Print and shaded views of the part. All mm, measured from the part's lowest x, y and z. A direction names the side the tool comes from. Give positions to 0.01 mm unless a question says otherwise; leave off trailing zeros. Loops run counter-clockwise (first coordinate to the right, second up) from the corner with the lowest first, then second, coordinate; pieces in that order, holes last. Notation, with made-up numbers: (66.25, 63) -> (78.25, 63) arc R25 cw to (78.25, 92) -> close; hole circle Ø6 at (32, 64). An arc over 180 degrees is marked (long way). Answer as a JSON object with one key per item and string values. Group by question number.
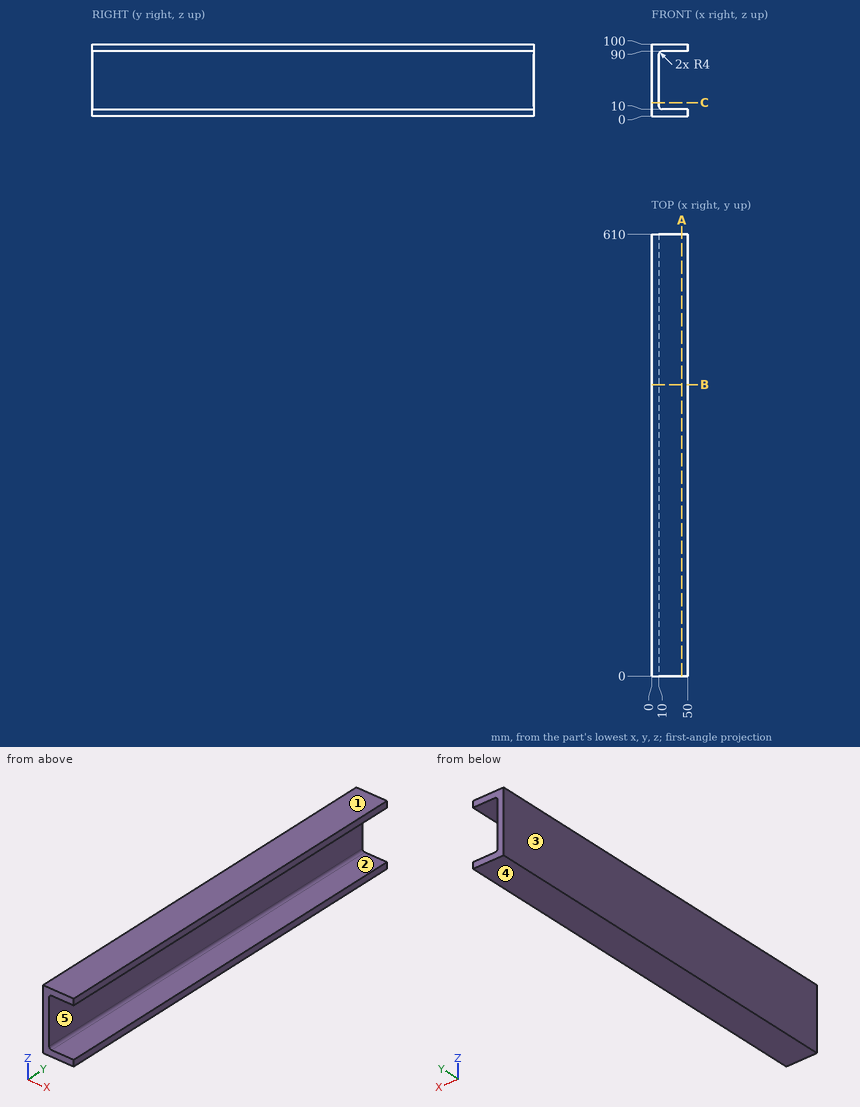
(1) Saw through at C-C on z = 19. List the corners of the cut face in (x, y).
(2) Pin check, flat tip, straight feed: pin 1 (21.5 mm diameter, centred on y = 414.5, z = 53.5, fed in from +X). Stop position of the tip, or through.
(3) Saw through at B-B on y = 402.5. List the corners of the cut face in (x, z), plus the area to 3 significant figures.
(4) 3-axis set-ups, long thin cutter, end or side, ignore diameter. For the marked faces 4 and 5: which of +Z, -Z, +X, -X, +Y, -Y reach the whole face in a straight line?
(5) Saw through at A-A on x = 41.5. List the corners of the cut face in (y, z).
(6) Probe line 1 along Z through (x, y) = (34, 397.5); line 2 along X through (y, z) = (340, 71); line 3 along Z through (x, y) = (13, 423). List the from-to ranges inside material, lowest first. Write a range as [from, to].
(7) Pull direction Z, two halves, no side cores. Call the marked faces 1, 2 and 3: pulls with the +Z half, pulls with the -Z half, needs draft (parallel to the pull), parting line crosses it, or undercut.
Calculated:
{
 "1": {"outline": "(0, 0) -> (10, 0) -> (10, 610) -> (0, 610) -> close"},
 "2": {"pin 1": "stops at x = 10"},
 "3": {"outline": "(0, 0) -> (50, 0) -> (50, 10) -> (14, 10) arc R4 cw to (10, 14) -> (10, 86) arc R4 cw to (14, 90) -> (50, 90) -> (50, 100) -> (0, 100) -> close", "area": "1,810 mm^2"},
 "4": {"face 4": "-Z, +X, -X, +Y, -Y", "face 5": "+X, +Y, -Y"},
 "5": {"outline": "(0, 0) -> (610, 0) -> (610, 10) -> (0, 10) -> close; (0, 90) -> (610, 90) -> (610, 100) -> (0, 100) -> close"},
 "6": {"line 1": "z = [0, 10], [90, 100]", "line 2": "x = [0, 10]", "line 3": "z = [0, 10.13], [89.87, 100]"},
 "7": {"face 1": "pulls with the +Z half", "face 2": "undercut", "face 3": "needs draft"}
}
